```python
from build123d import *

# Parameters (mm, degrees)
SKETCH1_R           = 4
BOSS_EXTRUDE1_DEPTH = 7
SKETCH2_R           = 5.5
BOSS_EXTRUDE2_DEPTH = 1
SKETCH3_R           = 9.525
BOSS_EXTRUDE3_DEPTH = 25.4
SKETCH4_R           = 6.35
CUT_EXTRUDE1_DEPTH  = 19.05
SKETCH5_R           = 1.5875
CUT_EXTRUDE2_DEPTH  = 25.4
CIRPATTERN1_COUNT   = 3


with BuildPart() as part:
    # Sketch1 → Boss-Extrude1 (new body)
    with BuildSketch(Plane.XY):
        Circle(SKETCH1_R)
    extrude(amount=BOSS_EXTRUDE1_DEPTH)

    # Sketch2 → Boss-Extrude2 (add)
    with BuildSketch(Plane.XY.offset(7)):
        Circle(SKETCH2_R)
    extrude(amount=BOSS_EXTRUDE2_DEPTH)

    # Sketch3 → Boss-Extrude3 (add)
    with BuildSketch(Plane.XY.offset(8)):
        Circle(SKETCH3_R)
    extrude(amount=BOSS_EXTRUDE3_DEPTH)

    # Sketch4 → Cut-Extrude1 (cut)
    with BuildSketch(Plane.XY.offset(33.4)):
        Circle(SKETCH4_R)
    extrude(amount=-CUT_EXTRUDE1_DEPTH, mode=Mode.SUBTRACT)

    # Sketch5 → Cut-Extrude2 (cut)
    with BuildSketch(Plane(origin=(0, 0, 0), x_dir=(1, 0, 0), z_dir=(0, 1, 0))):
        with Locations(Location((0, -27.05, 0), (0, 0, 270))):
            Circle(SKETCH5_R)
    cut_extrude2 = extrude(amount=-CUT_EXTRUDE2_DEPTH, mode=Mode.SUBTRACT)

    # CirPattern1: Cut-Extrude2 ×3 about axis
    cirpattern1_axis = Axis((0, 0, 33.4), (0, 0, -1))
    for i in range(1, CIRPATTERN1_COUNT):
        add(cut_extrude2.rotate(cirpattern1_axis, i * 360 / CIRPATTERN1_COUNT), mode=Mode.SUBTRACT)


solid = part.part
```
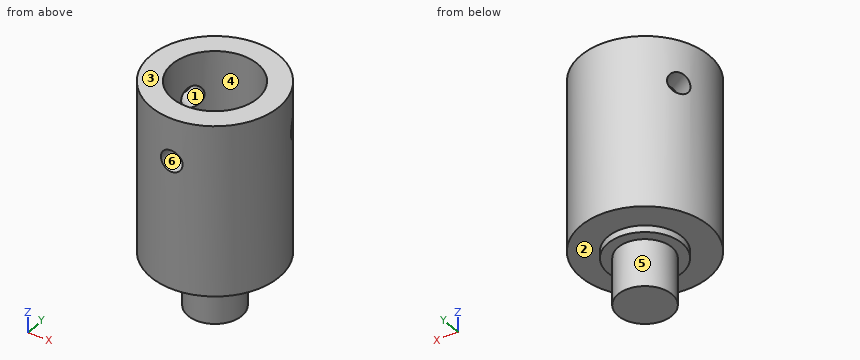
Build history of the part. All positions in model axes, mm. Face numbers are marked on the shaded views. A direction names the side the tool comes from. Give positions to 0.01 mm unless a question says otherwise; leave off trailing zeros. Order: outer loops, then holes, each group sorted by start corner. A loop starts at its lowest first (then second) coordinate and runs counter-clockwise, first axis right, second up. Notation, with made-up numbers: M -30.75,50.5 L 21.25,50.5 A13 cw 21.25,56.5 Z; hole C 45.5,76 d9. An arc over 180 degrees is marked long. Write item = value, one per line. Start each with the question number.
(1) Two-plate mould, pull along X, no slides. Class the marked faces 3, 4, 5 and 6: released by +X, released by -X, zero draft, split by the parting line, or undercut.
(2) Slice it at C-C on y = 0. Write the cut outline in (x, z) (3 decimals).
(3) Slice it at B-B on z = 27.05. State how many separate pieces and enclosed holes the cut face has, plus the area to 3 significant figures.
(4) Which spindle directions (+Z, -Z, +X, -X, +Y, -Y) get a long thin tool onto all of the face, cutting with end or side? Do the marked faces 1 and 2. Say none if no direction does.
(5) Probe L1, parallel to Y at x = 0, z = 19.25 (3 decimals); L2, parallel to Z at x = 0, y = -8.2; L3, parallel to Z at x = 6.25, y = -4.75. List the from-to ranges inside material, lowest first. Write a range as [from, to].
(6) Pin check, flat tips, straight feed: pin 1 Ø3 at (x, z) = (7, 9) entering from +Y; pin 2 Ø3 at (x, z) = (2, 4) entering from +Y; pin 3 Ø6.5 at (x, y) = (-2.5, 1) entering from +Z. Stop position of each tip, or through.
Responses:
q1.face_3 = zero draft
q1.face_4 = undercut
q1.face_5 = split by the parting line
q1.face_6 = undercut
q2.outline = M -9.525,8 L -5.5,8 L -5.5,7 L -4,7 L -4,0 L 4,0 L 4,7 L 5.5,7 L 5.5,8 L 9.525,8 L 9.525,33.4 L 6.35,33.4 L 6.35,14.35 L -6.35,14.35 L -6.35,33.4 L -9.525,33.4 Z
q3.separate_pieces = 3
q3.enclosed_holes = 0
q3.area = 128 mm2
q4.face_1 = none
q4.face_2 = -Z
q5.L1 = [-9.525, -6.35], [6.35, 9.525]
q5.L2 = [8, 25.46], [28.64, 33.4]
q5.L3 = [8, 33.4]
q6.pin_1 = 7.78
q6.pin_2 = 3.97
q6.pin_3 = 14.35
